from build123d import *

# Parameters (mm, degrees)
F0_W      = 65
F0_H      = 65
F1_DEPTH  = 350
F3_DEPTH  = 65.001
F4_W      = 75
F4_H      = 65
F5_DEPTH  = 2
F6_W      = 65
F6_H      = 75
F7_DEPTH  = 2
F10_DEPTH = 65.001


with BuildPart() as f1:
    # F0 (on Top) → F1 (new body)
    with BuildSketch(Plane.XY):
        Rectangle(F0_W, F0_H)
    extrude(amount=F1_DEPTH)

    # F2 (on face) → F3 (cut, through all)
    with BuildSketch(Plane.XZ.offset(32.5)):
        Polygon((-22.5, 175), (32.5, 120), (32.5, 230), align=None)
        Polygon((-32.5, 180), (-32.5, 170), (-27.5, 175), align=None)
    extrude(amount=-F3_DEPTH, mode=Mode.SUBTRACT)

    # F9 (on face) → F10 (cut, through all)
    with BuildSketch(Plane.XZ.offset(32.5)):
        Polygon((-32.5, 180), (-27.5, 175), (-22.5, 175), (32.5, 230), (32.5, 350), (-32.5, 350), align=None)
    extrude(amount=-F10_DEPTH, mode=Mode.SUBTRACT)


with BuildPart() as f5:
    # F4 (on face) → F5 (new body)
    with BuildSketch(Plane(origin=(76.25, 0, 76.25), x_dir=(0.7071067812, 0, -0.7071067812), z_dir=(0.7071067812, 0, 0.7071067812))):
        with Locations((-99.3718433538, 0)):
            Rectangle(F4_W, F4_H)
    extrude(amount=F5_DEPTH)


with BuildPart() as f7:
    # F6 (on face) → F7 (new body)
    with BuildSketch(Plane(origin=(-98.75, 0, 98.75), x_dir=(0, 1, 0), z_dir=(0.7071067812, 0, -0.7071067812))):
        with Locations((0, 148.1155300615)):
            Rectangle(F6_W, F6_H)
    extrude(amount=F7_DEPTH)


solid = f1.part
Can you work these out from the model? Positions are in its coordinate system, mm. Give positions to 0.01 mm unless a question says otherwise; leave off trailing zeros. Loops run counter-clockwise (first coordinate to the right, second up) from the corner with the lowest first, then second, coordinate; pieces in that order, holes last. Notation, with made-up numbers: M 64,53 L 80,53 A12 ccw 80,72 Z; hole C 33,65 d11. An arc over 180 degrees is marked long. One line per item, written item: value. Start each with the question number.
1) If I drill on line 1 (X direction, y = 2, z = 138); line 2 (Z direction, x = 3, y = 10.5); line 3 (Z direction, x = 17, y = -22), over which ranges is the centre line in solid material (lowest first)? Write a range as [from, to].
2) Thinking about a two-plate mould opening in Z: for faces 1 (the face through (0, 0, 0)), 2 (the face through (-25, 0, 175)), 3 (the face through (32.5, 0, 59)), which applies, +Z half, -Z half, draft (parallel to the pull), parting line (faces both ways), or undercut?
3) I'm going to push flat-ended pins straight in: pin 1 (4 mm diameter, centred on y = -10.5, z = 123, fed in from +X); pin 2 (2 mm diameter, centred on y = 13.5, z = 145.5, fed in from +X); pin 3 (12 mm diameter, centred on x = 22, y = -22.5, fed in from -Z); pin 4 (2 mm diameter, centred on y = -11, z = 155.5, fed in from +X). Where does each tip first touch, or does it pass through?
4) If we section it at A-A, the plane x = 18.5: Write out the boundary of the cut face in (y, z).
5) If we section it at B-B, the plane y = -9: Write out the boundary of the cut face in (x, z), and give its area (3 significant figures).
6) If we section it at C-C, the plane z = 135.5: Write out the boundary of the cut face in (x, y).
Completed:
1. line 1: x = [-32.5, 14.5]
1. line 2: z = [0, 149.5]
1. line 3: z = [0, 135.5]
2. face 1: -Z half
2. face 2: +Z half
2. face 3: draft
3. pin 1: stops at x = 31.5
3. pin 2: stops at x = 8
3. pin 3: stops at z = 0
3. pin 4: stops at x = -2
4. outline: M -32.5,0 L 32.5,0 L 32.5,134 L -32.5,134 Z
5. outline: M -32.5,0 L 32.5,0 L 32.5,120 L -22.5,175 L -27.5,175 L -32.5,170 Z
5. area: 9,850 mm^2
6. outline: M -32.5,-32.5 L 17,-32.5 L 17,32.5 L -32.5,32.5 Z
